from build123d import *

# Parameters (mm, degrees)
BOSS_EXTRUDE1_DEPTH     = 70
SKETCH2_W               = 100
SKETCH2_H               = 100
BOSS_EXTRUDE2_DEPTH     = 2
SKETCH3_W               = 6.255686465
SKETCH3_H               = 19
SKETCH3_R               = 1.5
SKETCH3_W_2             = 6.249842205
BOSS_EXTRUDE4_DEPTH     = 28
CUT_EXTRUDE2_DEPTH      = 49
CUT_EXTRUDE2_DEPTH_BACK = 10
SKETCH4_W               = 14.879207683
SKETCH4_H               = 12.351519759
SKETCH5_W               = 96.00443459
SKETCH5_H               = 43.693152777
BOSS_EXTRUDE5_DEPTH     = 2
SKETCH9_W               = 100
SKETCH9_H               = 100
CUT_EXTRUDE3_DEPTH      = 42
BOSS_EXTRUDE6_DEPTH     = 2
SKETCH8_R               = 1.5
BOSS_EXTRUDE7_DEPTH     = 10
SKETCH11_W              = 10
SKETCH11_H              = 10
SKETCH11_R              = 1.5
BOSS_EXTRUDE8_DEPTH     = 5
SKETCH13_R              = 2
CUT_EXTRUDE4_DEPTH      = 10
CUT_EXTRUDE5_DEPTH      = 3
SKETCH16_R              = 4.002775558
CUT_EXTRUDE7_DEPTH      = 3


with BuildPart() as part:
    # Sketch1 → Boss-Extrude1 (new body)
    with BuildSketch(Plane.XY):
        Polygon((-47.671840355, 33.254988914), (-47.671840355, 35.254988914), (-49.667405765, 35.254988914), (-49.667405765, -64.745011086), (50.332594235, -64.745011086), (50.332594235, 35.254988914), (48.332594235, 35.254988914), (48.332594235, 33.254988914), (48.332594235, -62.745011086), (-47.671840355, -62.745011086), align=None)
    extrude(amount=BOSS_EXTRUDE1_DEPTH)

    # Sketch2 → Boss-Extrude2 (add)
    with BuildSketch(Plane(origin=(0, 0, 0), x_dir=(-1, 0, 0), z_dir=(0, 0, -1))):
        with Locations((-0.332594235, -14.745011086)):
            Rectangle(SKETCH2_W, SKETCH2_H)
    extrude(amount=BOSS_EXTRUDE2_DEPTH)

    # Sketch3 → Boss-Extrude4 (add)
    # profile 1 of 2: a face of its own
    with BuildSketch(Plane.XY):
        with Locations((37.062045054, -23.882996664)):
            Rectangle(SKETCH3_W, SKETCH3_H)
        with Locations((37.169542955, -19.02966579)):
            Circle(SKETCH3_R, mode=Mode.SUBTRACT)
        with Locations((37.189888286, -28.916071788)):
            Circle(SKETCH3_R, mode=Mode.SUBTRACT)
    # profile 2 of 2: a face of its own
    with BuildSketch(Plane.XY):
        with Locations((-10.777585785, -23.882996664)):
            Rectangle(SKETCH3_W_2, SKETCH3_H)
        with Locations((-10.805764952, -18.882996664)):
            Circle(SKETCH3_R, mode=Mode.SUBTRACT)
        with Locations((-10.830457045, -29.02966579)):
            Circle(SKETCH3_R, mode=Mode.SUBTRACT)
    extrude(amount=BOSS_EXTRUDE4_DEPTH)

    # Sketch4 → Cut-Extrude2 (cut, two sides: drawn at the far end of the back side and taken through both)
    with BuildSketch(Plane.ZY.offset(-33.934201821).offset(-CUT_EXTRUDE2_DEPTH_BACK)):
        with Locations((10.28647213, -23.707236785)):
            Rectangle(SKETCH4_W, SKETCH4_H)
    extrude(amount=CUT_EXTRUDE2_DEPTH + CUT_EXTRUDE2_DEPTH_BACK, mode=Mode.SUBTRACT)

    # Sketch5 → Boss-Extrude5 (add)
    with BuildSketch(Plane.XY.offset(70)):
        with Locations((0.33037694, -40.898434698)):
            Rectangle(SKETCH5_W, SKETCH5_H)
    extrude(amount=-BOSS_EXTRUDE5_DEPTH)

    # Sketch9 → Cut-Extrude3 (cut)
    with BuildSketch(Plane(origin=(0, 0, 58), x_dir=(-1, 0, 0), z_dir=(0, 0, -1))):
        with Locations((-0.332594235, -14.745011086)):
            Rectangle(SKETCH9_W, SKETCH9_H)
    extrude(amount=-CUT_EXTRUDE3_DEPTH, mode=Mode.SUBTRACT)

    # Sketch10 → Boss-Extrude6 (add)
    with BuildSketch(Plane.XY.offset(58)):
        with BuildLine():
            Line((-49.667405765, -64.745011086), (50.332594235, -64.745011086))
            Line((50.332594235, -64.745011086), (50.332594235, -23.515098033))
            Line((50.332594235, -23.515098033), (16.092202794, -23.515098033))
            Line((16.092202794, -23.515098033), (5.242138191, -23.515098033))
            Line((5.242138191, -23.515098033), (5.242138191, -34.745011086))
            ThreePointArc((5.242138191, -34.745011086), (-2.857861809, -42.845011086), (-10.957861809, -34.745011086))
            Line((-10.957861809, -34.745011086), (-10.957861809, -23.515098033))
            Line((-10.957861809, -23.515098033), (-15.769437358, -23.515098033))
            Line((-15.769437358, -23.515098033), (-49.667405765, -23.515098033))
            Line((-49.667405765, -23.515098033), (-49.667405765, -64.745011086))
        make_face()
    extrude(amount=-BOSS_EXTRUDE6_DEPTH)

    # Sketch8 → Boss-Extrude7 (add)
    # profile 1 of 2: a face of its own
    with BuildSketch(Plane(origin=(0, 35.254988914, 0), x_dir=(1, 0, 0), z_dir=(0, 1, 0))):
        with BuildLine():
            Line((-47.671840355, 0), (-40.671840355, 0))
            ThreePointArc((-40.671840355, 0), (-42.722092886, -4.949747468), (-47.671840355, -7))
            Line((-47.671840355, -7), (-47.671840355, 0))
        make_face()
        with Locations(Location((-44.671840355, -3, 0), (0, 0, 270))):
            Circle(SKETCH8_R, mode=Mode.SUBTRACT)
    # profile 2 of 2: a face of its own
    with BuildSketch(Plane(origin=(0, 35.254988914, 0), x_dir=(1, 0, 0), z_dir=(0, 1, 0))):
        with BuildLine():
            Line((48.332594235, 0), (48.332594235, -7))
            ThreePointArc((48.332594235, -7), (43.382846767, -4.949747468), (41.332594235, 0))
            Line((41.332594235, 0), (48.332594235, 0))
        make_face()
        with Locations(Location((45.332594235, -3, 0), (0, 0, 270))):
            Circle(SKETCH8_R, mode=Mode.SUBTRACT)
    extrude(amount=-BOSS_EXTRUDE7_DEPTH)

    # Sketch11 → Boss-Extrude8 (add)
    # profile 1 of 2: a face of its own
    with BuildSketch(Plane.XY.offset(58)):
        with Locations((-54.667405765, 27.254988914)):
            Rectangle(SKETCH11_W, SKETCH11_H)
        with Locations((-54.949444375, 28.754988914)):
            Circle(SKETCH11_R, mode=Mode.SUBTRACT)
    # profile 2 of 2: a face of its own
    with BuildSketch(Plane.XY.offset(58)):
        with Locations((55.332594235, 27.254988914)):
            Rectangle(SKETCH11_W, SKETCH11_H)
        with Locations((55.832594235, 28.754988914)):
            Circle(SKETCH11_R, mode=Mode.SUBTRACT)
    extrude(amount=-BOSS_EXTRUDE8_DEPTH)

    # Sketch13 → Cut-Extrude4 (cut)
    with BuildSketch(Plane.XY.offset(58)):
        with Locations((-10.957861809, -29.13005456)):
            Circle(SKETCH13_R)
        with Locations((37.169542955, -29.02966579)):
            Circle(SKETCH13_R)
    extrude(amount=-CUT_EXTRUDE4_DEPTH, mode=Mode.SUBTRACT)

    # Sketch15 → Cut-Extrude5 (cut)
    with BuildSketch(Plane(origin=(0, 35.254988914, 0), x_dir=(1, 0, 0), z_dir=(0, 1, 0))):
        with BuildLine():
            Line((-47.671840355, -58), (-47.671840355, -7))
            ThreePointArc((-47.671840355, -7), (-42.722092886, -4.949747468), (-40.671840355, 0))
            Line((-40.671840355, 0), (41.332594235, 0))
            ThreePointArc((41.332594235, 0), (43.382846767, -4.949747468), (48.332594235, -7))
            Line((48.332594235, -7), (48.332594235, -58))
            Line((48.332594235, -58), (50.332594235, -58))
            Line((50.332594235, -58), (50.332594235, 2))
            Line((50.332594235, 2), (-49.667405765, 2))
            Line((-49.667405765, 2), (-49.667405765, -58))
            Line((-49.667405765, -58), (-47.671840355, -58))
        make_face()
    extrude(amount=-CUT_EXTRUDE5_DEPTH, mode=Mode.SUBTRACT)

    # Sketch16 → Cut-Extrude7 (cut)
    with BuildSketch(Plane(origin=(0, -62.745011086, 0), x_dir=(1, 0, 0), z_dir=(0, 1, 0))):
        with Locations(Location((44.016753305, -11.905726119, 0), (0, 0, 270))):
            Circle(SKETCH16_R)
    extrude(amount=-CUT_EXTRUDE7_DEPTH, mode=Mode.SUBTRACT)


solid = part.part
Work out the finished part from the listing and answer in its coordinate system (mm). A direction names the side the tool comes from. Give positions to 0.01 mm unless a question says otherwise; leave off trailing zeros. Loops run counter-clockwise (first coordinate to the right, second up) from the corner with the lowest first, then second, coordinate; pieces in that order, holes last. Notation, with made-up numbers: (-34, 82.25) - (11, 82.25) arc R22 cw to (11, 100.25) - close; hole circle Ø1 at (-2.75, -27.75). An arc over 180 degrees is marked (long way). Answer in a Markdown table with one row per item. Add a question column.
Q1. A tool of negligible diameter and unlimited length cuts with its end or side. For faces 1 (the cylindrical face through (-11.156, -30.494, 16.915)), 2 (the flat face through (0, -43, 56)), 3 (the flat face through (1, -15, 0)), 4 (the flat face through (55, 22.255, 56)), 5 (the cylindrical face through (-42.668, 28.804, 4.895)), from which of +Z, -Z, +X, -X, +Y, -Y can it reach the whole face along a straight path? Write none if from no direction.
Q2. Each of these flat-tipped pins is pushed along its axis until it touches: P1, Ø8, axis at y = -7, z = 8, coming from the -X side; P2, Ø7, axis at x = 37.5, z = 8.5, coming from the +Y side; P3, Ø1.8, axis at x = 37.19, y = -28.92, coming from the +Z side. Where does it stop, or does it pass through?
Q3. Determine the mould class of faces 6 (the flat face through (40.19, -24, 20)), 7 (the flat face through (37, -19, 0)), 8 (the flat face through (-7.653, -24, 20)) for opening direction Z: released by +Z, released by -Z, zero draft, split by the parting line, or undercut.
Q4. The part is cut by section A-A (y = -22). Determine the outline of the cut face in (x, z).
Q5. The part is cut by section B-B (z = 36.5). Determine the outline of the cut face in (x, y), and give its area (3 significant figures).
Q6. The part is cut by section D-D (x = 7). Determine the outline of the cut face in (y, z).
Q7. The part is cut by section C-C (y = -53). Determine the outline of the cut face in (x, z).
Q8. Consider line 1 along X through (y, z) = (-1.5, 44.5); line 2 along X through (y, z) = (30, 3); line 3 along Y through (x, z) = (-39, 30). Determine where each line is inside the solid, lowest interval first.
Solution:
| question | item | result |
|---|---|---|
| 1 | face 1 | +Z |
| 1 | face 2 | +Y |
| 1 | face 3 | none |
| 1 | face 4 | +Z, -Z, +X, -Y |
| 1 | face 5 | +Z, +Y |
| 2 | P1 | stops at x = -49.67 |
| 2 | P2 | stops at y = -14.38 |
| 2 | P3 | stops at z = 0 |
| 3 | face 6 | undercut |
| 3 | face 7 | released by +Z |
| 3 | face 8 | zero draft |
| 4 | outline | (-49.67, -2) - (50.33, -2) - (50.33, 58) - (48.33, 58) - (48.33, 0) - (40.19, 0) - (40.19, 2.85) - (33.93, 2.85) - (33.93, 0) - (-7.65, 0) - (-7.65, 2.85) - (-13.9, 2.85) - (-13.9, 0) - (-47.67, 0) - (-47.67, 58) - (-49.67, 58) - close; (-13.9, 17.73) - (-7.65, 17.73) - (-7.65, 28) - (-13.9, 28) - close; (33.93, 17.73) - (40.19, 17.73) - (40.19, 28) - (33.93, 28) - close |
| 5 | outline | (-49.67, -64.75) - (50.33, -64.75) - (50.33, 32.25) - (48.33, 32.25) - (48.33, -62.75) - (-47.67, -62.75) - (-47.67, 32.25) - (-49.67, 32.25) - close |
| 5 | area | 580 mm² |
| 6 | outline | (-64.75, -2) - (32.25, -2) - (32.25, 0) - (-62.75, 0) - (-62.75, 56) - (-23.52, 56) - (-23.52, 58) - (-64.75, 58) - close |
| 7 | outline | (-49.67, -2) - (50.33, -2) - (50.33, 58) - (-49.67, 58) - close; hole (-47.67, 0) - (48.33, 0) - (48.33, 56) - (-47.67, 56) - close |
| 8 | line 1 | x = -49.67 to -47.67, 48.33 to 50.33 |
| 8 | line 2 | x = -49.67 to -46.17, -43.17 to -41.35, 42.01 to 43.83, 46.83 to 50.33 |
| 8 | line 3 | y = -64.75 to -62.75 |
